Check sheet for the modelled part. Datum: model origin and axes. Units: mm. A direction names the side the tool comes from. Give positions to 0.01 mm unless a question says otherwise; leave off trailing zeros. Order: outer loops, then holes, each group sorted by start corner. A loop starts at its lowest first (then second) coordinate and runs counter-clockwise, first axis right, second up. Notation, with made-up numbers: (30.5, -12) - (37.5, -12) arc R38 cw to (37.5, 26) - close; hole circle Ø9 at (88, -20). An arc over 180 degrees is marked (long way). Answer in a Markdown table with one row per item.
from build123d import *

# Parameters (mm, degrees)
SKETCH1_W           = 317.5
SKETCH1_H           = 317.5
SKETCH1_W_2         = 266.7
SKETCH1_H_2         = 266.7
BOSS_EXTRUDE1_DEPTH = 25.4
SKETCH2_W           = 304.8
SKETCH2_H           = 304.8
BOSS_EXTRUDE2_DEPTH = 6.35
SKETCH3_R           = 127
BOSS_EXTRUDE3_DEPTH = 23.876
SKETCH4_R           = 86.741
CUT_EXTRUDE1_DEPTH  = 56.626


with BuildPart() as part:
    # Sketch1 → Boss-Extrude1 (new body)
    with BuildSketch(Plane(origin=(0, 0, 0), x_dir=(1, 0, 0), z_dir=(0, 1, 0))):
        Rectangle(SKETCH1_W, SKETCH1_H)
        Rectangle(SKETCH1_W_2, SKETCH1_H_2, mode=Mode.SUBTRACT)
    extrude(amount=BOSS_EXTRUDE1_DEPTH)

    # Sketch2 → Boss-Extrude2 (add)
    with BuildSketch(Plane(origin=(0, 25.4, 0), x_dir=(1, 0, 0), z_dir=(0, 1, 0))):
        Rectangle(SKETCH2_W, SKETCH2_H)
    extrude(amount=BOSS_EXTRUDE2_DEPTH)

    # Sketch3 → Boss-Extrude3 (add)
    with BuildSketch(Plane(origin=(0, 31.75, 0), x_dir=(1, 0, 0), z_dir=(0, 1, 0))):
        Circle(SKETCH3_R)
    extrude(amount=BOSS_EXTRUDE3_DEPTH)

    # Sketch4 → Cut-Extrude1 (cut, through all)
    with BuildSketch(Plane(origin=(0, 55.626, 0), x_dir=(1, 0, 0), z_dir=(0, 1, 0))):
        Circle(SKETCH4_R)
    extrude(amount=-CUT_EXTRUDE1_DEPTH, mode=Mode.SUBTRACT)


solid = part.part
(1) Cross-section at B-B, the plane z = 0. Record the cut outline in (x, y).
Geometry says:
| item | result |
|---|---|
| outline | (-158.75, 0) - (-133.35, 0) - (-133.35, 25.4) - (-86.74, 25.4) - (-86.74, 55.63) - (-127, 55.63) - (-127, 31.75) - (-152.4, 31.75) - (-152.4, 25.4) - (-158.75, 25.4) - close; (86.74, 25.4) - (133.35, 25.4) - (133.35, 0) - (158.75, 0) - (158.75, 25.4) - (152.4, 25.4) - (152.4, 31.75) - (127, 31.75) - (127, 55.63) - (86.74, 55.63) - close |
(2) Access from +Z, -Z, +X, -X, +Y, -Y to the whole of each face (thin tool, end or side, straight path). Record for faces 5 (the flat face through (-138, 31.75, -2)), 6 (the flat face through (83, 55.626, 26)), 7 (the flat face through (-2, 13, -133.35)).
Geometry says:
| item | result |
|---|---|
| face 5 | +Y |
| face 6 | +Z, -Z, +X, -X, +Y |
| face 7 | -Y |
(3) Cross-section at C-C, the plane z = -113.5. Record the cut outline in (x, y), then the cut area to 3 significant figures.
Geometry says:
| item | result |
|---|---|
| outline | (-158.75, 0) - (-133.35, 0) - (-133.35, 25.4) - (133.35, 25.4) - (133.35, 0) - (158.75, 0) - (158.75, 25.4) - (152.4, 25.4) - (152.4, 31.75) - (56.98, 31.75) - (56.98, 55.63) - (-56.98, 55.63) - (-56.98, 31.75) - (-152.4, 31.75) - (-152.4, 25.4) - (-158.75, 25.4) - close |
| area | 5,950 mm² |
(4) Cross-section at D-D, the plane x = -98.5. Record the cut outline in (y, z), then the cut area to 3 significant figures.
Geometry says:
| item | result |
|---|---|
| outline | (0, -158.75) - (25.4, -158.75) - (25.4, -152.4) - (31.75, -152.4) - (31.75, -80.17) - (55.63, -80.17) - (55.63, 80.17) - (31.75, 80.17) - (31.75, 152.4) - (25.4, 152.4) - (25.4, 158.75) - (0, 158.75) - (0, 133.35) - (25.4, 133.35) - (25.4, -133.35) - (0, -133.35) - close |
| area | 7,050 mm² |
(5) Gauge pin test, flat ends, axial feed: P1, Ø7, axis at x = 61.5, y = 29.5, coming from the +Z side; P2, Ø7, axis at y = 29.5, z = -59.5, coming from the -X side; P3, Ø1.9, axis at x = -18, y = 29.5, coming from the -Z side. Record the tip position at first contact, or that the pin passes through.
Geometry says:
| item | result |
|---|---|
| P1 | z = 152.4 |
| P2 | x = -152.4 |
| P3 | z = -152.4 |
(6) Cross-section at A-A, the plane x = 0. Record the cut outline in (y, z).
Geometry says:
| item | result |
|---|---|
| outline | (0, -158.75) - (25.4, -158.75) - (25.4, -152.4) - (31.75, -152.4) - (31.75, -127) - (55.63, -127) - (55.63, -86.74) - (25.4, -86.74) - (25.4, -133.35) - (0, -133.35) - close; (0, 133.35) - (25.4, 133.35) - (25.4, 86.74) - (55.63, 86.74) - (55.63, 127) - (31.75, 127) - (31.75, 152.4) - (25.4, 152.4) - (25.4, 158.75) - (0, 158.75) - close |
(7) Thickness scan on L1, parallel to X at y = 16.5, z = 92; L2, parallel to X at y = 40, z = 0. Record the ranges inside material, lowest first.
Geometry says:
| item | result |
|---|---|
| L1 | -158.75 to -133.35, 133.35 to 158.75 |
| L2 | -127 to -86.74, 86.74 to 127 |
(8) Mould release check, pull along Z, two halves, no side actions. Record for faces 1 (the cylindrical face through (-27.53, 43.52, 123.98)), 2 (the flat face through (-158.75, 13, 2)), 3 (the flat face through (133.35, 13, 2)), 4 (the flat face through (-2, 13, 158.75)): pulls with the +Z half, pulls with the -Z half, needs draft (parallel to the pull), parting line crosses it, or undercut.
Geometry says:
| item | result |
|---|---|
| face 1 | parting line crosses it |
| face 2 | needs draft |
| face 3 | undercut |
| face 4 | pulls with the +Z half |
